Geometry: final body of the model. Coordinates: model frame, mm. A direction names the side the tool comes from. Give positions to 0.01 mm unless a question says otherwise; leave off trailing zeros. Write each loop counter-clockwise with the first axis right and the second up, starting at its lowest first coordinate (ties: lowest second). Pieces come first, ordered by that corner, then holes.
Q1. Section C-C (y = -3.5). Return the cut outline in (x, z).
Q2. Reachability of faces 5 (the cylindrical face through (-34.666, -87.089, 0.022)), 6 (the flat face through (43.068, -90.576, 0.022)) from +Z, -Z, +X, -X, +Y, -Y: full face, straight path, thin tool, end or side. Return the list, or none.
Q3. Section A-A (x = -22). State how many separate pieces and enclosed holes the cut face has, plus the area to 3 significant figures.
Q4. Section B-B (z = 0.85). Return the cut outline in (x, y) (3 decimals), plus the area to 3 significant figures.
Q5. Section D-D (y = 64.5). Return the cut outline in (x, z), plus the area to 3 significant figures.
Q6. Mould query, pull axis X, two halves, no side actions, for faces 1 (the cylindrical face through (-34.765, 86.99, 0.022)), 2 (the flat face through (20.923, -72.803, 0.022)), 3 (the flat face through (42.062, 91.582, 0.022)), 4 (the flat face through (-51, 2, -1.588)). Classes: +X half, -X half, draft (parallel to the pull), parting line (faces both ways), or undercut.
Q7. Line query: line 1 (X direction, y = -4.5, z = -1.2); line 2 (Y direction, x = -4.5, z = -1); line 3 (Y direction, x = 30.5, z = 0). Output: solid intervals per line, ascending.
from build123d import *

# Parameters (mm, degrees)
SKETCH1_W         = 25.4
SKETCH1_H         = 3.175
PLATE_DEPTH       = 1.5875
CENTER_HOLE_DEPTH = 150.328941672


with BuildPart() as part:
    # Sketch1 → Plate (new, symmetric)
    with BuildSketch(Plane.XY):
        Polygon((-78.486, 127), (6.643951031, 127), (78.486, 55.157951031), (78.486, -55.157951031), (6.643951031, -127), (-78.486, -127), align=None)
        with Locations((-27.686, 122.2375)):
            Rectangle(SKETCH1_W, SKETCH1_H, mode=Mode.SUBTRACT)
        with Locations((-27.686, -122.2375)):
            Rectangle(SKETCH1_W, SKETCH1_H, mode=Mode.SUBTRACT)
    extrude(amount=PLATE_DEPTH, both=True)

    # Sketch4 → Center Hole (cut, through all)
    with BuildSketch(Plane.XY.offset(1.5875)):
        with BuildLine():
            Line((4.826, 88.9), (36.576, 57.15))
            Line((36.576, 57.15), (36.576, -57.15))
            Line((36.576, -57.15), (4.826, -88.9))
            Line((4.826, -88.9), (-30.226, -88.9))
            ThreePointArc((-30.226, -88.9), (-34.716128061, -87.040128061), (-36.576, -82.55))
            Line((-36.576, -82.55), (-36.576, 82.55))
            ThreePointArc((-36.576, 82.55), (-34.716128061, 87.040128061), (-30.226, 88.9))
            Line((-30.226, 88.9), (4.826, 88.9))
        make_face()
    extrude(amount=-CENTER_HOLE_DEPTH, mode=Mode.SUBTRACT)


solid = part.part
Computed:
1. outline: (-78.49, -1.59) - (-36.58, -1.59) - (-36.58, 1.59) - (-78.49, 1.59) - close; (36.58, -1.59) - (78.49, -1.59) - (78.49, 1.59) - (36.58, 1.59) - close
2. face 5: +Z, -Z
2. face 6: +Z, -Z, +X, -Y
3. separate pieces: 4
3. enclosed holes: 0
3. area: 222 mm2
4. outline: (-78.486, -127) - (6.644, -127) - (78.486, -55.158) - (78.486, 55.158) - (6.644, 127) - (-78.486, 127) - close; hole (-40.386, -123.825) - (-14.986, -123.825) - (-14.986, -120.65) - (-40.386, -120.65) - close; hole (-40.386, 120.65) - (-14.986, 120.65) - (-14.986, 123.825) - (-40.386, 123.825) - close; hole (-36.576, -82.55) arc R6.35 ccw to (-30.226, -88.9) - (4.826, -88.9) - (36.576, -57.15) - (36.576, 57.15) - (4.826, 88.9) - (-30.226, 88.9) arc R6.35 ccw to (-36.576, 82.55) - close
4. area: 22,600 mm2
5. outline: (-78.49, -1.59) - (-36.58, -1.59) - (-36.58, 1.59) - (-78.49, 1.59) - close; (29.23, -1.59) - (69.14, -1.59) - (69.14, 1.59) - (29.23, 1.59) - close
5. area: 260 mm2
6. face 1: undercut
6. face 2: undercut
6. face 3: +X half
6. face 4: draft
7. line 1: x = -78.49 to -36.58, 36.58 to 78.49
7. line 2: y = -127 to -88.9, 88.9 to 127
7. line 3: y = -103.14 to -63.23, 63.23 to 103.14
